Verification items for the finished model (mm, model axes). Face numbers are marked on the shaded views. Round coordinates to 2 decimals unless told otherwise and drop trailing zeros. Loops run counter-clockwise (first coordinate to the right, second up) from the corner with the lowest first, then second, coordinate; pieces in that order, holes last. Notation, with made-up numbers: M 32,-2.75 L 42,-2.75 A19 ccw 42,6.25 Z; hole C 64.5,8.25 d10. An arc over 180 degrees is marked long. One line per item, written item: value.
from build123d import *


with BuildPart() as part:
    # Szkic1 → Obrót1 (revolve)
    with BuildSketch(Plane.XY, mode=Mode.PRIVATE) as obr_t1_sk:
        with BuildLine():
            Line((-23.04, -50.853493976), (-23.04, 55.146506024))
            Line((-23.04, 55.146506024), (-23.02, 55.146506024))
            ThreePointArc((-23.02, 55.146506024), (-20.191572875, 53.974933149), (-19.02, 51.146506024))
            Line((-19.02, 51.146506024), (-19.02, -41.145145612))
            ThreePointArc((-19.02, -41.145145612), (-18.757277337, -41.820735819), (-18.107155743, -42.14134031))
            Line((-18.107155743, -42.14134031), (-9.51, -42.893493976))
            Line((-9.51, -42.893493976), (0, -42.893493976))
            Line((0, -42.893493976), (0, -51.853493976))
            Line((0, -51.853493976), (-22.04, -51.853493976))
            ThreePointArc((-22.04, -51.853493976), (-22.747106781, -51.560600757), (-23.04, -50.853493976))
        make_face()
    revolve(obr_t1_sk.sketch.rotate(Axis((0, -51.853493976, 0), (0, 1, 0)), 180), axis=Axis((0, -51.853493976, 0), (0, 1, 0)))


solid = part.part
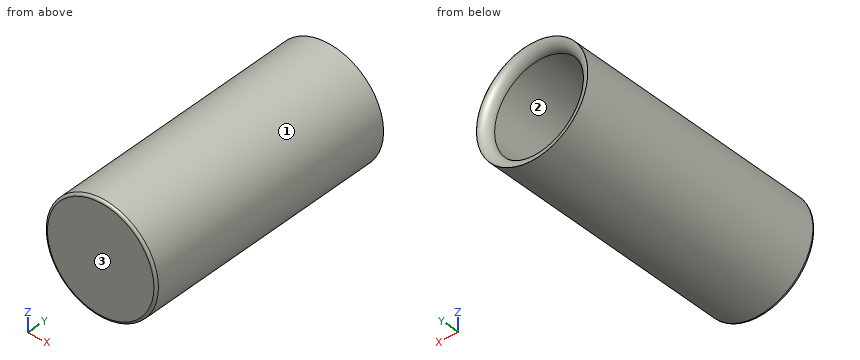
(1) Sectioned sample at C-C on y = -12.5. Enter the section's corners in (x, z).
Completed:
outline: C 0,0 d46.08; hole C 0,0 d38.04
(2) Thickness scan on L1, parallel to Z at x = 0, y = -8.5; L2, parallel to Y at x = -3.5, z = 1.5; L3, parallel to Z at x = 16, y = -17.5. Record the ranges inside material, lowest first. Write a range as from..to.
Completed:
L1: z = -23.04..-19.02, 19.02..23.04
L2: y = -51.85..-42.89
L3: z = -16.58..-10.28, 10.28..16.58
(3) Depth check by flat-ended pin: pin 1 Ø1 at (x, y) = (9, -27) entering from -Z; pin 2 Ø5.5 at (x, z) = (-2, -3.5) entering from +Y; pin 3 Ø10 at (x, z) = (16.5, -2.5) entering from +Y. Enter the tip coordinate at first touch or a pass-through.
Completed:
pin 1: stops at z = -21.41
pin 2: stops at y = -42.89
pin 3: stops at y = 54.92
(4) Mould release check, pull along X, two halves, no side actions. Record for the marked faces 1, 2 and 3: +X half, -X half, draft (parallel to the pull), parting line (faces both ways), or undercut.
Completed:
face 1: parting line
face 2: undercut
face 3: draft
